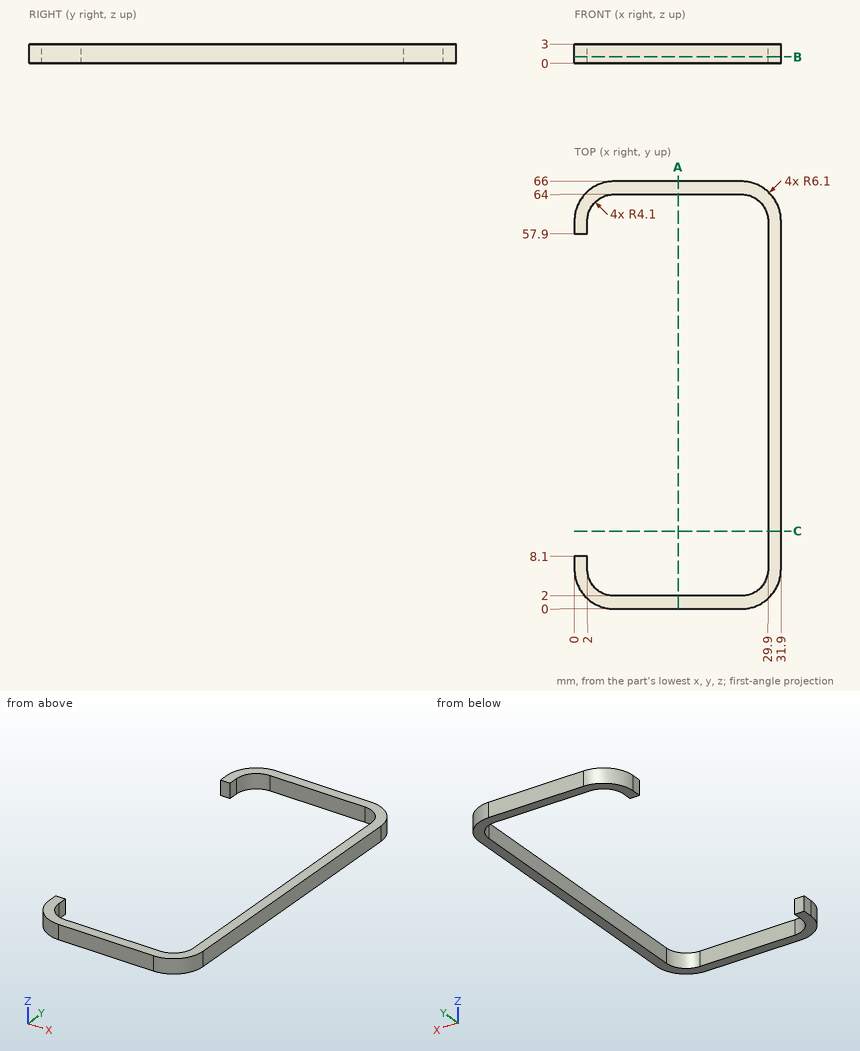
Here's the drawing with two shaded views (mm, measured from the low corner). I have some questions. Coordinates: 2 decimals unless noted, no trailing zeros. Order: outer loops, then holes, each group sorted by start corner. A loop starts at its lowest first (then second) coordinate and runs counter-clockwise, first axis right, second up.
Item 1: I need wall thicknesses on line 1 (Y direction, x = 22.5, z = 0.7); line 2 (X direction, y = 8, z = 2.7); line 3 (X direction, y = 13, z = 2.45). Which ranges of each line are inside material? Lowest first, please.
Result sheet:
line 1: y = 0 to 2, 64 to 66
line 2: x = 0 to 2, 29.9 to 31.9
line 3: x = 29.9 to 31.9
Item 2: If we section it at C-C on y = 12: List the corners of the cut face in (x, z) for me.
Result sheet:
outline: (29.9, 0) - (31.9, 0) - (31.9, 3) - (29.9, 3) - close
Item 3: If we section it at A-A on x = 16: List the corners of the cut face in (y, z) for me.
Result sheet:
outline: (0, 0) - (2, 0) - (2, 3) - (0, 3) - close; (64, 0) - (66, 0) - (66, 3) - (64, 3) - close
Item 4: For P1, Ø1.6, axis at x = 1.5, z = 1, coming from the +Y side, with a flat end and sliding along its axis, tell me the tip position at first contact or that it passes through.
Result sheet:
P1: stops at y = 64.67
Item 5: If we section it at B-B on z = 1: List the corners of the cut face in (x, y) for me, plus the area to 3 significant figures.
Result sheet:
outline: (0, 6.1) arc R6.1 ccw to (6.1, 0) - (25.8, 0) arc R6.1 ccw to (31.9, 6.1) - (31.9, 59.9) arc R6.1 ccw to (25.8, 66) - (6.1, 66) arc R6.1 ccw to (0, 59.9) - (0, 57.9) - (2, 57.9) - (2, 59.9) arc R4.1 cw to (6.1, 64) - (25.8, 64) arc R4.1 cw to (29.9, 59.9) - (29.9, 6.1) arc R4.1 cw to (25.8, 2) - (6.1, 2) arc R4.1 cw to (2, 6.1) - (2, 8.1) - (0, 8.1) - close
area: 258 mm2
